Work out the finished part from the listing and answer in its coordinate system (mm). Round coordinates to 2 decimals unless told otherwise and drop trailing zeros. Write each loop counter-clockwise with the first axis right and the second up, starting at its lowest first coordinate (ties: lowest second). Pieces come first, ordered by that corner, then holes. Notation, with made-up numbers: M 31.25,12 L 55.25,12 A29 cw 55.25,40 Z; hole C -31,54 d11. An arc over 180 degrees is marked long. One line per item, written item: value. Start each with the question number.
Q1. Find section B-B (x = 75). Write down the section's boundary in (y, z), and give its area (3 significant figures).
Q2. Consider probe 1 along Y at (x, z) = (-89.5, 2.45); probe 2 along X at (y, z) = (-64, 1.2); probe 3 along Y at (x, z) = (-98, 0.4). Determine where each line is inside the solid, lowest interval first.
Q3. Find section C-C (z = 2). Count the separate pieces of the cut face and the enclosed holes in it, and give its area (3 significant figures).
Q4. Find section A-A (y = -82.5). Write down the section's boundary in (x, z).
Autodesk Inventor part; units mm, degrees
ref_plane "YZ Plane" through (0, 0, 0) normal (1, 0, 0) x (0, 1, 0)
ref_plane "XZ Plane" through (0, 0, 0) normal (0, 1, 0) x (-1, 0, 0)
ref_plane "XY Plane" through (0, 0, 0) normal (0, 0, 1) x (1, 0, 0)
sketch "Эскиз1" plane through (0, 0, 0) normal (0, 0, 1) x (1, 0, 0)
  line L0 (-149.5, 116.5) -> (149.5, 116.5)
  line L1 (164.5, 101.5) -> (164.5, -101.5)
  line L2 (149.5, -116.5) -> (-149.5, -116.5)
  line L3 (-164.5, -101.5) -> (-164.5, 101.5)
  line L4 (0, -167.4492) -> (0, 167.4492)
  line L5 (-234.6492, 0) -> (234.6492, 0)
  arc A0 (-149.5, 116.5) -> (-164.5, 101.5) centre (-149.5, 101.5) ccw
  arc A1 (164.5, 101.5) -> (149.5, 116.5) centre (149.5, 101.5) ccw
  arc A2 (149.5, -116.5) -> (164.5, -101.5) centre (149.5, -101.5) ccw
  arc A3 (-164.5, -101.5) -> (-149.5, -116.5) centre (-149.5, -101.5) ccw
  circle A4 centre (-154.5, 106.5) radius 1.35
  circle A5 centre (154.5, 106.5) radius 1.35
  circle A6 centre (154.5, -106.5) radius 1.35
  circle A7 centre (-154.5, -106.5) radius 1.35
  point P0 (0, 0)
  dimension "d0" = 329
  dimension "d1" = 233
  dimension "d2" = 15
  dimension "d3" = 2.7
  dimension "d4" = 2.7
  dimension "d5" = 2.7
  dimension "d6" = 2.7
  dimension "d7" = 5
  dimension "d8" = 5
  dimension "d9" = 5
  dimension "d10" = 5
  dimension "d11" = 5
  dimension "d12" = 5
  dimension "d13" = 5
  dimension "d14" = 5
extrude "Выдавливание1" add sketch "Эскиз1" along normal blind 3
sketch "Эскиз2" plane through (0, 0, 3) normal (0, 0, 1) x (1, 0, 0)
  line L0 (149.5, 110.5) -> (59.5, 110.5)
  line L1 (59.5, 110.5) -> (59.5, -111.5)
  line L2 (59.5, -111.5) -> (149.5, -111.5)
  line L3 (149.5, -111.5) -> (149.5, 110.5)
  line L4 (54.5, 110.5) -> (-15.5, 110.5)
  line L5 (-15.5, 110.5) -> (-15.5, -111.5)
  line L6 (-15.5, -111.5) -> (54.5, -111.5)
  line L7 (54.5, -111.5) -> (54.5, 110.5)
  line L8 (-20.5, 110.5) -> (-80.5, 110.5)
  line L9 (-80.5, 110.5) -> (-80.5, -111.5)
  line L10 (-80.5, -111.5) -> (-20.5, -111.5)
  line L11 (-20.5, -111.5) -> (-20.5, 110.5)
  circle A0 centre (154.5, 106.5) radius 1.35
  line L12 (-85.5, 110.5) -> (-150.85, 110.5)
  line L13 (-150.85, 110.5) -> (-150.85, -111.5)
  line L14 (-150.85, -111.5) -> (-85.5, -111.5)
  line L15 (-85.5, -111.5) -> (-85.5, 110.5)
  circle A1 centre (-154.5, 106.5) radius 1.35
  line L16 (-149.5, -116.5) -> (149.5, -116.5)
  line L17 (149.5, 116.5) -> (-149.5, 116.5)
  line L18 (-145.85, 106.5) -> (-90.5, 106.5)
  line L19 (-90.5, 106.5) -> (-90.5, -106.5)
  line L20 (-90.5, -106.5) -> (-145.85, -106.5)
  line L21 (-145.85, -106.5) -> (-145.85, 106.5)
  line L22 (-75.5, 106.5) -> (-25.5, 106.5)
  line L23 (-25.5, 106.5) -> (-25.5, -106.5)
  line L24 (-25.5, -106.5) -> (-75.5, -106.5)
  line L25 (-75.5, -106.5) -> (-75.5, 106.5)
  line L26 (-10.5, 106.5) -> (49.5, 106.5)
  line L27 (49.5, 106.5) -> (49.5, -106.5)
  line L28 (49.5, -106.5) -> (-10.5, -106.5)
  line L29 (-10.5, -106.5) -> (-10.5, 106.5)
  line L30 (64.5, 106.5) -> (144.5, 106.5)
  line L31 (144.5, 106.5) -> (144.5, -106.5)
  line L32 (144.5, -106.5) -> (64.5, -106.5)
  line L33 (64.5, -106.5) -> (64.5, 106.5)
  point P0 (0, 0)
  point P1 (19.5, -106.5)
  dimension "d18" = 70
  dimension "d19" = 60
  dimension "d20" = 5
  dimension "d21" = 5
  dimension "d22" = 5
  dimension "d23" = 90
  dimension "d25" = 5
  dimension "d26" = 5
  dimension "d27" = 5
  dimension "d29" = 6
  dimension "d30" = 4
  dimension "d31" = 5
  dimension "d32" = 5
  dimension "d33" = 5
  dimension "d34" = 5
  dimension "d35" = 5
  dimension "d36" = 5
  dimension "d37" = 5
  dimension "d38" = 5
  dimension "d39" = 5
  dimension "d40" = 5
  dimension "d41" = 5
  dimension "d42" = 5
extrude "Выдавливание2" cut sketch "Эскиз2" against normal blind 3 contours L18 L19 L20 L21 | L22 L23 L24 L25 | L26 L27 L28 L29 | L30 L31 L32 L33
sketch "Эскиз3" plane through (0, 0, 3) normal (0, 0, 1) x (1, 0, 0)
  circle A0 centre (-146.85, 107.5) radius 1.35
  circle A1 centre (-89.5, 107.5) radius 1.35
  circle A2 centre (-146.85, -107.5) radius 1.35
  circle A3 centre (-89.5, -107.5) radius 1.35
  line L0 (-145.85, -106.5) -> (-145.85, 106.5)
  line L1 (-145.85, 106.5) -> (-90.5, 106.5)
  line L2 (-90.5, 106.5) -> (-90.5, -106.5)
  line L3 (-90.5, -106.5) -> (-145.85, -106.5)
  circle A4 centre (-76.5, -107.5) radius 1.35
  circle A5 centre (-24.5, -107.5) radius 1.35
  circle A6 centre (-76.5, 107.5) radius 1.35
  circle A7 centre (-24.5, 107.5) radius 1.35
  circle A8 centre (-11.5, 107.5) radius 1.35
  circle A9 centre (-11.5, -107.5) radius 1.35
  circle A10 centre (50.5, -107.5) radius 1.35
  circle A11 centre (50.5, 107.5) radius 1.35
  line L4 (-75.5, -106.5) -> (-75.5, 106.5)
  line L5 (-75.5, 106.5) -> (-25.5, 106.5)
  line L6 (-25.5, 106.5) -> (-25.5, -106.5)
  line L7 (-25.5, -106.5) -> (-75.5, -106.5)
  line L8 (-10.5, -106.5) -> (-10.5, 106.5)
  line L9 (-10.5, 106.5) -> (49.5, 106.5)
  line L10 (49.5, 106.5) -> (49.5, -106.5)
  line L11 (49.5, -106.5) -> (-10.5, -106.5)
  circle A12 centre (63.5, 107.5) radius 1.35
  circle A13 centre (63.5, -107.5) radius 1.35
  circle A14 centre (145.5, -107.5) radius 1.35
  circle A15 centre (145.5, 107.5) radius 1.35
  line L12 (64.5, -106.5) -> (64.5, 106.5)
  line L13 (64.5, 106.5) -> (144.5, 106.5)
  line L14 (144.5, 106.5) -> (144.5, -106.5)
  line L15 (144.5, -106.5) -> (64.5, -106.5)
  point P0 (0, 0)
  dimension "d45" = 2.7
  dimension "d46" = 2.7
  dimension "d47" = 2.7
  dimension "d48" = 2.7
  dimension "d49" = 1
  dimension "d51" = 1
  dimension "d52" = 1
  dimension "d53" = 1
  dimension "d54" = 1
  dimension "d55" = 1
  dimension "d56" = 1
  dimension "d57" = 1
  dimension "d58" = 2.7
  dimension "d59" = 2.7
  dimension "d60" = 2.7
  dimension "d61" = 2.7
  dimension "d62" = 2.7
  dimension "d63" = 2.7
  dimension "d64" = 2.7
  dimension "d65" = 2.7
  dimension "d66" = 1
  dimension "d67" = 1
  dimension "d68" = 1
  dimension "d69" = 1
  dimension "d70" = 1
  dimension "d71" = 1
  dimension "d72" = 1
  dimension "d73" = 1
  dimension "d74" = 1
  dimension "d75" = 1
  dimension "d76" = 1
  dimension "d77" = 1
  dimension "d78" = 1
  dimension "d79" = 1
  dimension "d80" = 1
  dimension "d81" = 1
  dimension "d82" = 2.7
  dimension "d83" = 2.7
  dimension "d84" = 2.7
  dimension "d85" = 2.7
  dimension "d86" = 1
  dimension "d87" = 1
  dimension "d88" = 1
  dimension "d89" = 1
  dimension "d90" = 1
  dimension "d91" = 1
  dimension "d92" = 1
  dimension "d93" = 1
extrude "Выдавливание3" cut sketch "Эскиз3" against normal blind 10 contours A0 | A1 | A2 | A3 | A4 | A5 | A6 | A7 | A8 | A9 | A10 | A11 | A12 | A13 | A14 | A15
fillet "Сопряжение1" radius 2 1 edges at (64.5, 106.5, 1.5)
fillet "Сопряжение2" radius 2 5 edges at (144.5, 106.5, 1.5) (64.5, -106.5, 1.5) (144.5, -106.5, 1.5) (49.5, -106.5, 1.5) (-10.5, -106.5, 1.5)
fillet "Сопряжение3" radius 2 6 edges at (-10.5, 106.5, 1.5) (49.5, 106.5, 1.5) (-25.5, 106.5, 1.5) (-75.5, 106.5, 1.5) (-25.5, -106.5, 1.5) (-75.5, -106.5, 1.5)
fillet "Сопряжение4" radius 2 4 edges at (-145.85, -106.5, 1.5) (-90.5, -106.5, 1.5) (-90.5, 106.5, 1.5) (-145.85, 106.5, 1.5)
properties part number "рамка насу"
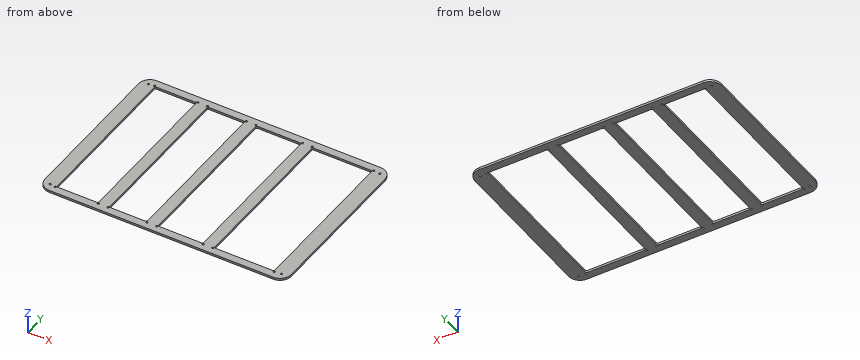
The answers:
1. outline: M -116.5,0 L -106.5,0 L -106.5,3 L -116.5,3 Z; M 106.5,0 L 116.5,0 L 116.5,3 L 106.5,3 Z
1. area: 60.0 mm2
2. probe 1: -116.5 to -108.85, -106.15 to 106.15, 108.85 to 116.5
2. probe 2: -164.5 to -145.85, -90.5 to -75.5, -25.5 to -10.5, 49.5 to 64.5, 144.5 to 164.5
2. probe 3: -116.5 to -106.5, 106.5 to 116.5
3. separate pieces: 1
3. enclosed holes: 24
3. area: 24,100 mm2
4. outline: M -164.5,0 L -145.85,0 L -145.85,3 L -164.5,3 Z; M -90.5,0 L -75.5,0 L -75.5,3 L -90.5,3 Z; M -25.5,0 L -10.5,0 L -10.5,3 L -25.5,3 Z; M 49.5,0 L 64.5,0 L 64.5,3 L 49.5,3 Z; M 144.5,0 L 164.5,0 L 164.5,3 L 144.5,3 Z
